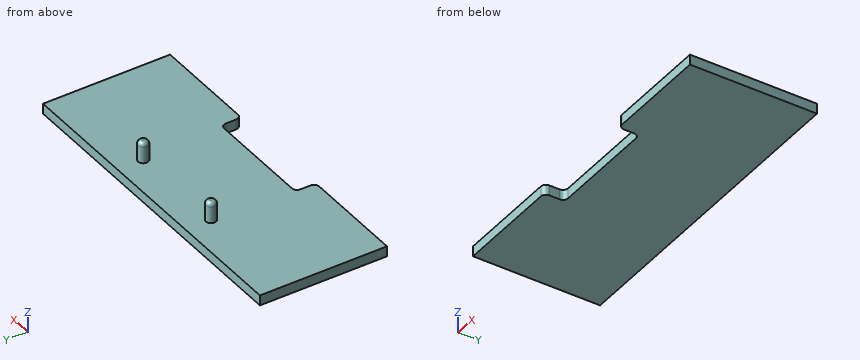
```python
from build123d import *

# Parameters (mm, degrees)
SKETCH1_W           = 203.2
SKETCH1_H           = 78.7146
BOSS_EXTRUDE1_DEPTH = 6.35
SKETCH2_W           = 69.85
SKETCH2_H           = 12.7
CUT_EXTRUDE1_DEPTH  = 219.005850273
FILLET1_R           = 3.175
SKETCH3_R           = 3.175
BOSS_EXTRUDE2_DEPTH = 12.7
FILLET2_R           = 2.38125


with BuildPart() as part:
    # Sketch1 → Boss-Extrude1 (new body)
    with BuildSketch(Plane.XY):
        with Locations((101.6, 39.3573)):
            Rectangle(SKETCH1_W, SKETCH1_H)
    extrude(amount=BOSS_EXTRUDE1_DEPTH)

    # Sketch2 → Cut-Extrude1 (cut, through all)
    with BuildSketch(Plane.XY.offset(6.35)):
        with Locations((101.6, 6.35)):
            Rectangle(SKETCH2_W, SKETCH2_H)
    extrude(amount=-CUT_EXTRUDE1_DEPTH, mode=Mode.SUBTRACT)

    # Fillet1
    fillet1_edges = [part.edges().sort_by_distance(p)[0] for p in [
        (66.675, 0, 3.175),
        (66.675, 12.7, 3.175),
        (136.525, 12.7, 3.175),
        (136.525, 0, 3.175),
    ]]
    fillet(fillet1_edges, radius=FILLET1_R)

    # Sketch3 → Boss-Extrude2 (add)
    with BuildSketch(Plane.XY.offset(6.35)):
        with Locations(Location((69.85, 62.8396, 0), (0, 0, 180))):
            Circle(SKETCH3_R)
        with Locations(Location((133.35, 62.8396, 0), (0, 0, 180))):
            Circle(SKETCH3_R)
    extrude(amount=BOSS_EXTRUDE2_DEPTH)

    # Fillet2
    fillet2_edges = [part.edges().sort_by_distance(p)[0] for p in [
        (73.025, 62.8396, 19.05),
        (136.525, 62.8396, 19.05),
    ]]
    fillet(fillet2_edges, radius=FILLET2_R)


solid = part.part
```
Here's how the part is built. I have some questions about the finished solid (model axes, mm). Round coordinates to 2 decimals unless told otherwise and drop trailing zeros. Order: outer loops, then holes, each group sorted by start corner. A loop starts at its lowest first (then second) coordinate and runs counter-clockwise, first axis right, second up. Notation, with made-up numbers: (18, -17) -> (25, -17) arc R24 cw to (25, 4) -> close; hole circle Ø7 at (10.25, 17). An arc over 180 degrees is marked (long way). Use a Markdown table: item, result. Add a question column.
(1) Suppose I cut it at C-C, the plane y = 26. Please give me the cut outline in (x, z), and give its area (3 significant figures).
(2) I need wall thicknesses on line 1 along X through (y, z) = (5.5, 5.5) (3 decimals); line 2 along Z through (x, y) = (82, 14); line 3 along X through (y, z) = (60.5, 7.5). Which ranges of each line are inside material? Lowest first, please.
(3) Suppose I cut it at A-A, the plane z = 4.5. Please give me the cut outline in (x, y) (3 decimals).
(4) Suppose I cut it at D-D, the plane z = 14.25. Please give me the cut outline in (x, y) (3 decimals), and give its area (3 significant figures).
(5) Suppose I cut it at B-B, the plane x = 41. Please give me the cut outline in (y, z), and give its area (3 significant figures).
(6) For pin 1 Ø6 at (x, y) = (173, 65.5) entering from +Z; pin 2 Ø3 at (x, z) = (116, 3.5) entering from -Y, each with a flat end and sliding along its axis, tell me the tip position at first contact or that it passes through.
Verdict:
| question | item | result |
|---|---|---|
| 1 | outline | (0, 0) -> (203.2, 0) -> (203.2, 6.35) -> (0, 6.35) -> close |
| 1 | area | 1,290 mm2 |
| 2 | line 1 | 0 to 66.675, 136.525 to 203.2 |
| 2 | line 2 | 0 to 6.35 |
| 2 | line 3 | 67.7 to 72, 131.2 to 135.5 |
| 3 | outline | (0, 0) -> (63.5, 0) arc R3.175 ccw to (66.675, 3.175) -> (66.675, 9.525) arc R3.175 cw to (69.85, 12.7) -> (133.35, 12.7) arc R3.175 cw to (136.525, 9.525) -> (136.525, 3.175) arc R3.175 ccw to (139.7, 0) -> (203.2, 0) -> (203.2, 78.715) -> (0, 78.715) -> close |
| 4 | outline | circle Ø6.35 at (69.85, 62.84); circle Ø6.35 at (133.35, 62.84) |
| 4 | area | 63.3 mm2 |
| 5 | outline | (0, 0) -> (78.71, 0) -> (78.71, 6.35) -> (0, 6.35) -> close |
| 5 | area | 500 mm2 |
| 6 | pin 1 | z = 6.35 |
| 6 | pin 2 | y = 12.7 |
